Autodesk Inventor part; units mm, degrees
ref_plane "YZ Plane" through (0, 0, 0) normal (1, 0, 0) x (0, 1, 0)
ref_plane "XZ Plane" through (0, 0, 0) normal (0, 1, 0) x (-1, 0, 0)
ref_plane "XY Plane" through (0, 0, 0) normal (0, 0, 1) x (1, 0, 0)
sketch "Sketch1" plane through (0, 0, 0) normal (0, 1, 0) x (-1, 0, 0)
  line L0 (-45, -75) -> (45, -75)
  line L1 (45, -75) -> (45, 75)
  line L2 (45, 75) -> (-45, 75)
  line L3 (-45, 75) -> (-45, -75)
  line L4 (-45, -75) -> (45, 75) construction
  line L5 (45, -75) -> (-45, 75) construction
  point P0 (0, 0)
  dimension "d0" = 150
  dimension "d1" = 90
extrude "Extrusion1" add sketch "Sketch1" along normal blind 6.35
chamfer "Chamfer1" distance 3.175 angle 45 4 edges at (45, 6.35, 0) (0, 6.35, 75) (-45, 6.35, 0) (0, 6.35, -75)
sketch "Sketch3" plane through (0, 6.35, 0) normal (0, 1, 0) x (1, 0, 0)
  line L0 (-45, -75) -> (45, -75)
  line L1 (-45, 75) -> (-45, -75)
  line L2 (45, -75) -> (45, 75)
  line L3 (45, 75) -> (-45, 75)
  point P0 (0, 0)
  point P1 (-35.4, -67)
  point P2 (-35.4, 67)
  point P3 (32.4, 67)
  point P4 (32.4, -67)
  dimension "d7" = 9.6
  dimension "d8" = 8
  dimension "d9" = 8
  dimension "d10" = 12.6
hole "Hole1" at (-35.4, 6.35, 67) at (-35.4, 6.35, -67) at (32.4, 6.35, -67) at (32.4, 6.35, 67) direction (0, -1, 0) diameter 4.7 depth 7.9 tip angle 118 counterbore diameter 7.9 counterbore depth 4.4
sketch "Sketch4" plane through (0, 0, 0) normal (0, -1, 0) x (1, 0, 0)
  line L0 (45, -75) -> (-45, -75)
  point P0 (0, 0)
  point P1 (-33.75, -13.5)
  point P2 (-33.75, 13.5)
  point P3 (-20.25, 13.5)
  point P4 (-20.25, -13.5)
  point P5 (-6.75, 13.5)
  point P6 (-6.75, -13.5)
  point P7 (6.75, 13.5)
  point P8 (6.75, -13.5)
  point P9 (20.25, 13.5)
  point P10 (20.25, -13.5)
  point P11 (33.75, 13.5)
  point P12 (33.75, -13.5)
  dimension "d18" = 27
  dimension "d19" = 13.5
  dimension "d22" = 13.5
  dimension "d34" = 6.75
hole "Hole2" at (-33.75, 0, -13.5) at (-33.75, 0, 13.5) at (-20.25, 0, 13.5) at (-20.25, 0, -13.5) at (-6.75, 0, 13.5) at (-6.75, 0, -13.5) at (6.75, 0, 13.5) at (6.75, 0, -13.5) at (20.25, 0, 13.5) at (20.25, 0, -13.5) at (33.75, 0, 13.5) at (33.75, 0, -13.5) direction (0, 1, 0) diameter 4.5 depth 7.9 tip angle 118 countersink diameter 9.4 countersink angle 90
properties part number "Mounting Plate" material "Aluminum 6061"
The model under review builds one solid part; all positions refer to its coordinate system, in mm. A direction names the side the tool comes from. Coordinates: 2 decimals unless noted, no trailing zeros. Loops run counter-clockwise (first coordinate to the right, second up) from the corner with the lowest first, then second, coordinate; pieces in that order, holes last. Notation, with made-up numbers: (86.5, -13) -> (96.5, -13) arc R31 ccw to (96.5, 25) -> close; hole circle Ø2 at (19, 13). An arc over 180 degrees is marked (long way). Use a Markdown table: item, result. Add a question column.
1. Add section C-C on z = 23. Write out the cut boundary in (x, y) (3 decimals).
2. Clearance check with flat-ended pins moving along their axes: pin 1 Ø2.5 at (x, z) = (6.75, 13.5) entering from -Y; pin 2 Ø6 at (x, z) = (-35.4, -67) entering from +Y; pin 3 Ø3 at (y, z) = (5, 13.5) entering from -X (3 decimals); pin 4 Ø6 at (x, z) = (-20.25, -13.5) entering from -Y. State where each tip first meets the part, or that it passes through.
3. Machinability: for faces 1 (the face through (-6.64, 2.3, 15.9)), 2 (the face through (-32.996, 4.119, 63.865)), which of the approach directions +Z, -Z, +X, -X, +Y, -Y give a long, thin tool a straight path to every point of the face, cutting with its end or side? Answer none if there is none.
4. Draft analysis for pull direction Z (two halves, no side actions). For faces 3 (the face through (1, 2, -75)), 4 (the face through (43.39, 4.785, -1.05)), 5 (the face through (34.804, 4.119, -70.135)), state which applies: pulls with the +Z half, pulls with the -Z half, needs draft (parallel to the pull), parting line crosses it, or undercut.
5. Add section A-A on x = -20.25. Write out the cut boundary in (y, z) (3 decimals), plus the area to 3 significant figures.
6. To check wall thickness, follow line 1 (X direction, y = 0.85, z = -67); line 2 (Z direction, x = 19.5, y = 4.5) (3 decimals); line 3 (Z direction, x = -20.25, y = 3.45) (3 decimals). State the ranges of each line that lie inside material, in increasing order.
7. Add section B-B on z = 67. Write out the cut boundary in (x, y) (3 decimals).
Returned:
| question | item | result |
|---|---|---|
| 1 | outline | (-45, 0) -> (45, 0) -> (45, 3.175) -> (41.825, 6.35) -> (-41.825, 6.35) -> (-45, 3.175) -> close |
| 2 | pin 1 | passes through |
| 2 | pin 2 | stops at y = 1.95 |
| 2 | pin 3 | stops at x = -44.675 |
| 2 | pin 4 | stops at y = 1.7 |
| 3 | face 1 | -Y |
| 3 | face 2 | +Y |
| 4 | face 3 | pulls with the -Z half |
| 4 | face 4 | needs draft |
| 4 | face 5 | undercut |
| 5 | outline | (0, -75) -> (3.175, -75) -> (6.35, -71.825) -> (6.35, -15.75) -> (2.45, -15.75) -> (0, -18.2) -> close; (0, -8.8) -> (2.45, -11.25) -> (6.35, -11.25) -> (6.35, 11.25) -> (2.45, 11.25) -> (0, 8.8) -> close; (0, 18.2) -> (2.45, 15.75) -> (6.35, 15.75) -> (6.35, 71.825) -> (3.175, 75) -> (0, 75) -> close |
| 5 | area | 873 mm² |
| 6 | line 1 | x = -45 to -37.75, -33.05 to 30.05, 34.75 to 45 |
| 6 | line 2 | z = -73.675 to -15.621, -11.379 to 11.379, 15.621 to 73.675 |
| 6 | line 3 | z = -74.725 to -15.75, -11.25 to 11.25, 15.75 to 74.725 |
| 7 | outline | (-45, 0) -> (-37.75, 0) -> (-37.75, 1.95) -> (-39.35, 1.95) -> (-39.35, 6.35) -> (-41.825, 6.35) -> (-45, 3.175) -> close; (-33.05, 0) -> (30.05, 0) -> (30.05, 1.95) -> (28.45, 1.95) -> (28.45, 6.35) -> (-31.45, 6.35) -> (-31.45, 1.95) -> (-33.05, 1.95) -> close; (34.75, 0) -> (45, 0) -> (45, 3.175) -> (41.825, 6.35) -> (36.35, 6.35) -> (36.35, 1.95) -> (34.75, 1.95) -> close |
